Work out the finished part from the listing and answer in its coordinate system (mm). A direction names the side the tool comes from. Coordinates: 2 decimals unless noted, no trailing zeros. Loops run counter-clockwise (first coordinate to the right, second up) from the corner with the lowest first, then second, coordinate; pieces in that order, holes last. Notation, with made-up numbers: (27.25, 20.25) -> (77.25, 20.25) arc R19 ccw to (77.25, 34.25) -> close; hole circle Ø5 at (71, 25). An arc over 180 degrees is marked (long way). Use a Markdown table: item, result.
from build123d import *

# Parameters (mm, degrees)
F1_DEPTH = 63.5
F2_DEPTH = 25.4
F3_DEPTH = 7.9375
F5_R     = 6.35


with BuildPart() as f1:
    # F0 (on Front) → F1 (new body, symmetric)
    with BuildSketch(Plane.XZ):
        Polygon((41.275, -9.525), (41.275, 9.525), (22.225, 9.525), (-41.275, 9.525), (-41.275, -9.525), align=None)
    extrude(amount=F1_DEPTH, both=True)

    # F0 (on Front) → F2 (join, symmetric)
    with BuildSketch(Plane.XZ):
        with BuildLine():
            Line((22.225, 9.525), (41.275, 9.525))
            Line((41.275, 9.525), (41.275, 27.0002))
            ThreePointArc((41.275, 27.0002), (45.92468, 38.22552), (57.15, 42.8752))
            Line((57.15, 42.8752), (66.177751, 42.8752))
            Line((66.177751, 42.8752), (66.177751, 61.9252))
            Line((66.177751, 61.9252), (57.15, 61.9252))
            ThreePointArc((57.15, 61.9252), (32.454296, 51.695904), (22.225, 27.0002))
            Line((22.225, 27.0002), (22.225, 9.525))
        make_face()
        Polygon((66.177751, 61.9252), (66.177751, 42.8752), (66.177751, 38.1), (116.977751, 38.1), (116.977751, 66.675), (66.177751, 66.675), align=None)
    extrude(amount=F2_DEPTH, both=True)

    # F0 (on Front) → F3 (join, symmetric)
    with BuildSketch(Plane.XZ):
        with BuildLine():
            Line((-41.275, 9.525), (22.225, 9.525))
            Line((22.225, 9.525), (22.225, 27.0002))
            ThreePointArc((22.225, 27.0002), (32.454296, 51.695904), (57.15, 61.9252))
            add(Edge.make_bspline(
                [(-41.275, 9.525), (-41.624442, 50.289135), (7.305516, 62.18183), (57.15, 61.9252)],
                knots=[0, 0, 0, 0, 111.504536, 111.504536, 111.504536, 111.504536], degree=3))
        make_face()
    extrude(amount=F3_DEPTH, both=True)

    # F0 (on Front) → F4 (revolve)
    with BuildSketch(Plane.XZ):
        Polygon((66.177751, 61.9252), (66.177751, 42.8752), (66.177751, 38.1), (116.977751, 38.1), (116.977751, 66.675), (66.177751, 66.675), align=None)
    revolve(axis=Axis((116.977751, 0, 52.3875), (0, 0, 1)))

    # F5
    f5_edges = [f1.edges().sort_by_distance(p)[0] for p in [
        (41.275, 63.5, 0),
        (41.275, -63.5, 0),
        (-41.275, -63.5, 0),
        (-41.275, 63.5, 0),
    ]]
    fillet(f5_edges, radius=F5_R)


solid = f1.part
Q1. Section C-C on x = 136.5 is taken. Determine the outline of the cut face in (y, z) (3 decimals).
Solved:
| item | result |
|---|---|
| outline | (-46.899, 38.1) -> (46.899, 38.1) -> (46.899, 66.675) -> (-46.899, 66.675) -> close |
Q2. Given pin 1 Ø10 at (x, y) = (59.5, -9.5) entering from +Z; pin 2 Ø4 at (y, z) = (35.5, 45) entering from +X; pin 3 Ø5 at (y, z) = (3.5, 65.5) entering from -X, each flat-ended and moving along its own axis, determine where each tip first touches the part or whether it passes through.
Solved:
| item | result |
|---|---|
| pin 1 | z = 61.93 |
| pin 2 | x = 155.17 |
| pin 3 | x = 66.18 |
Q3. Section B-B on y = -30 is taken. Determine the outline of the cut face in (x, z) (3 decimals), and give its area (3 significant figures).
Solved:
| item | result |
|---|---|
| outline | (-41.275, -9.525) -> (41.275, -9.525) -> (41.275, 9.525) -> (-41.275, 9.525) -> close; (75.982, 38.1) -> (157.973, 38.1) -> (157.973, 66.675) -> (75.982, 66.675) -> close |
| area | 3,920 mm² |
Q4. Consider line 1 (Z direction, x = -29.5, y = 25.5) (3 decimals); line 2 (Z direction, x = 99, y = 3.5) (3 decimals); line 3 (Y direction, x = 71, z = 51.5). Determine where each line is inside the solid, lowest interval first. Write a range as [from, to].
Solved:
| item | result |
|---|---|
| line 1 | [-9.525, 9.525] |
| line 2 | [38.1, 66.675] |
| line 3 | [-25.4, 25.4] |
Q5. Section D-D on x = 111.5 is taken. Determine the outline of the cut face in (y, z) (3 decimals), and give its area (3 significant figures).
Solved:
| item | result |
|---|---|
| outline | (-50.504, 38.1) -> (50.504, 38.1) -> (50.504, 66.675) -> (-50.504, 66.675) -> close |
| area | 2,890 mm² |
Q6. Section A-A on y = 36 is taken. Determine the outline of the cut face in (x, z) (3 decimals).
Solved:
| item | result |
|---|---|
| outline | (-41.275, -9.525) -> (41.275, -9.525) -> (41.275, 9.525) -> (-41.275, 9.525) -> close; (81.136, 38.1) -> (152.82, 38.1) -> (152.82, 66.675) -> (81.136, 66.675) -> close |
Q7. For faces 1 (the flat face through (22.225, -17, 18)), 2 (the cylindrical face through (45.8, -0.4, 38.1)), 3 (the flat face through (118, -1, 38.1)), determine the directions among +Z, -Z, +X, -X, +Y, -Y from which every point of the face is accessible in a straight line to the end or side of a thin tool.
Solved:
| item | result |
|---|---|
| face 1 | +Z, -X, -Y |
| face 2 | -Z, +Y, -Y |
| face 3 | -Z, +X, +Y, -Y |
